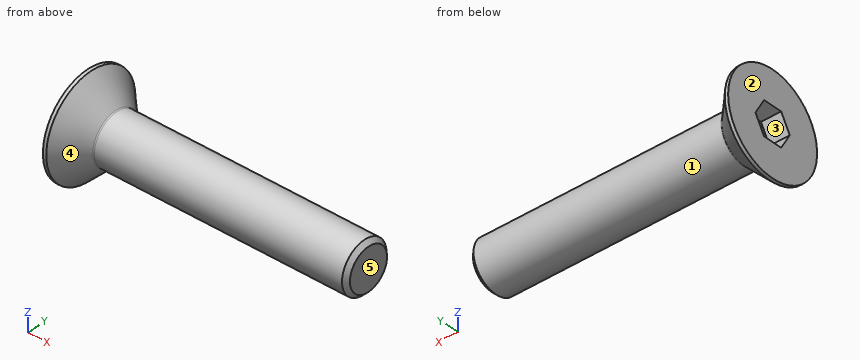
```python
from build123d import *

# Parameters (mm, degrees)
CUT_EXTRUDE_1_DEPTH = 1.2
CHAMFER_1_SIZE      = 0.25
FILLET_1_R          = 0.1


with BuildPart() as part:
    # 草圖1 → 旋轉1 (revolve)
    with BuildSketch(Plane.XY):
        Polygon((0, 3), (0, 0), (16.7, 0), (16.7, 1.5), (1.7, 1.5), (0.2, 3), align=None)
    revolve(axis=Axis((0, 0, 0), (1, 0, 0)))

    # 草圖2 → 除料-伸長1 (cut)
    with BuildSketch(Plane.ZY):
        Polygon((-1, -0.577350269), (0, -1.154700538), (1, -0.577350269), (1, 0.577350269), (0, 1.154700538), (-1, 0.577350269), align=None)
    extrude(amount=-CUT_EXTRUDE_1_DEPTH, mode=Mode.SUBTRACT)

    # 導角1
    chamfer_1_edges = [part.edges().sort_by_distance(p)[0] for p in [
        (16.7, -1.5, 0),
    ]]
    chamfer(chamfer_1_edges, length=CHAMFER_1_SIZE)

    # 圓角1
    fillet_1_edges = [part.edges().sort_by_distance(p)[0] for p in [
        (1.7, -1.5, 0),
    ]]
    fillet(fillet_1_edges, radius=FILLET_1_R)


solid = part.part
```
Verification items for the finished model (mm, model axes). Face numbers are marked on the shaded views. A direction names the side the tool comes from. Round coordinates to 2 decimals unless told otherwise and drop trailing zeros. Order: outer loops, then holes, each group sorted by start corner. A loop starts at its lowest first (then second) coordinate and runs counter-clockwise, first axis right, second up. Notation, with made-up numbers: (67, 80) - (75, 80) arc R32 cw to (75, 115) - close; hole circle Ø2 at (-9, 81). An arc over 180 degrees is marked (long way). Use CSV: the item, a comma, the result in double quotes. Start each with the question number.
1) Section check A-A, the plane x = 2.75. Record the cut outline in (y, z).
2) Access from +Z, -Z, +X, -X, +Y, -Y to the whole of each face (thin tool, end or side, straight path). Record for the marked faces 1 and 2.
3) Mould release check, pull along Z, two halves, no side actions. Record for the marked faces 3, 4 and 5: +Z half, -Z half, draft (parallel to the pull), parting line (faces both ways), or undercut.
4) Go/stop test with flat-tipped pins: P1, Ø2, axis at x = 8.5, y = 1, coming from the -Z side; P2, Ø1.5, axis at x = 8, z = -1.5, coming from the +Y side. Record where each tip stops, or that it passes through.
5) Thickness scan on L1, parallel to Z at x = 7.5, y = 0; L2, parallel to X at y = -0.5, z = 0.75; L3, parallel to X at y = 2.25, z = -1. Record the ranges inside material, lowest first.
Answers:
1,outline,"circle Ø3 at (0, 0)"
2,face 1,"+X"
2,face 2,"+Z, -Z, -X, +Y, -Y"
3,face 3,"undercut"
3,face 4,"parting line"
3,face 5,"draft"
4,P1,"stops at z = -1.5"
4,P2,"stops at y = 1.3"
5,L1,"z = -1.5 to 1.5"
5,L2,"x = 1.2 to 16.7"
5,L3,"x = 0 to 0.74"
